CAD build for the part. Positions are in the model's coordinates, mm. Face numbers are marked on the shaded views. Coordinates: 2 decimals unless noted, no trailing zeros. Order: outer loops, then holes, each group sorted by start corner. A loop starts at its lowest first (then second) coordinate and runs counter-clockwise, first axis right, second up. Notation, with made-up numbers: M -11.75,16 L 15.25,16 A20 ccw 15.25,42 Z; hole C 49.25,78 d2. An arc over 180 degrees is marked long. One line per item, written item: value.
from build123d import *

# Parameters (mm, degrees)
SKETCH_W             = 34.6
SKETCH_H             = 24.6
PAD001_DEPTH         = 1
SKETCH002_R          = 1.016
PAD002_DEPTH         = 5
LINEARPATTERN_COUNT  = 2
LINEARPATTERN_PITCH  = 17.9
SKETCH003_W          = 35.8
SKETCH003_H          = 25.8
PAD003_DEPTH         = 10
POCKET_DEPTH         = 12.901
POCKET_DEPTH_BACK    = 12.901
POCKET001_DEPTH      = 17.901
POCKET001_DEPTH_BACK = 17.901
SKETCH006_W          = 34.6
SKETCH006_H          = 24.6
POCKET002_DEPTH      = 2


with BuildPart() as digit001:
    # Sketch → Pad001 (new body)
    with BuildSketch(Plane.XY):
        Rectangle(SKETCH_W, SKETCH_H)
    extrude(amount=PAD001_DEPTH)

    # Sketch002 → Pad002 (join)
    with BuildSketch(Plane.XY):
        with Locations((-2.484719, -9.134)):
            Circle(SKETCH002_R)
        Polygon((-11.875322, 9.261), (-10.815853, 10.15), (-3.50471, 10.15), (-2.75875, 9.261), (-3.818219, 8.372), (-11.129362, 8.372), align=None)
        Polygon((-12.171581, 9.021337), (-11.425621, 8.132337), (-12.643997, 1.222585), (-13.703466, 0.333585), (-14.449425, 1.222585), (-13.23105, 8.132337), align=None)
        Polygon((-2.56357, 8.927415), (-3.623039, 8.038415), (-4.841415, 1.128663), (-4.095455, 0.239663), (-3.035986, 1.128663), (-1.81761, 8.038415), align=None)
        Polygon((-12.448817, 0.889), (-13.508286, 0), (-12.762326, -0.889), (-5.451183, -0.889), (-4.391714, 0), (-5.137674, 0.889), align=None)
        Polygon((-13.804545, -0.239663), (-14.864014, -1.128663), (-16.08239, -8.038415), (-15.33643, -8.927415), (-14.276961, -8.038415), (-13.058585, -1.128663), align=None)
        Polygon((-4.196534, -0.333585), (-5.256003, -1.222585), (-6.474379, -8.132337), (-5.728419, -9.021337), (-4.66895, -8.132337), (-3.450575, -1.222585), align=None)
        Polygon((-15.14125, -9.261), (-14.081781, -8.372), (-6.770638, -8.372), (-6.024678, -9.261), (-7.084147, -10.15), (-14.39529, -10.15), align=None)
    pad002 = extrude(amount=PAD002_DEPTH)

    # LinearPattern: Pad002 ×2
    with Locations(*[(i * LINEARPATTERN_PITCH, 0, 0) for i in range(1, LINEARPATTERN_COUNT)]):
        add(pad002)


with BuildPart() as digit001_1:
    # Body001 placement: moved
    add(digit001.part.moved(Location((0, 0, 5))))


with BuildPart() as obj1:
    # Sketch003 → Pad003 (new body)
    with BuildSketch(Plane.XY):
        Rectangle(SKETCH003_W, SKETCH003_H)
    extrude(amount=PAD003_DEPTH)

    # Sketch004 → Pocket (cut, two sides)
    with BuildSketch(Plane.XZ) as pocket_sk:
        Polygon((-16.9, 0), (-15.9, 1), (15.9, 1), (16.9, 0), align=None)
    extrude(amount=-POCKET_DEPTH, mode=Mode.SUBTRACT)
    extrude(pocket_sk.sketch, amount=POCKET_DEPTH_BACK, mode=Mode.SUBTRACT)

    # Sketch005 → Pocket001 (cut, two sides)
    with BuildSketch(Plane.YZ) as pocket001_sk:
        Polygon((-11.9, 0), (11.9, 0), (10.9, 1), (-10.9, 1), align=None)
    extrude(amount=-POCKET001_DEPTH, mode=Mode.SUBTRACT)
    extrude(pocket001_sk.sketch, amount=POCKET001_DEPTH_BACK, mode=Mode.SUBTRACT)

    # Sketch006 → Pocket002 (cut)
    with BuildSketch(Plane.XY):
        Rectangle(SKETCH006_W, SKETCH006_H)
    extrude(amount=POCKET002_DEPTH, mode=Mode.SUBTRACT)

    # Cut: cut Digit001
    add(digit001_1.part, mode=Mode.SUBTRACT)


solid = obj1.part
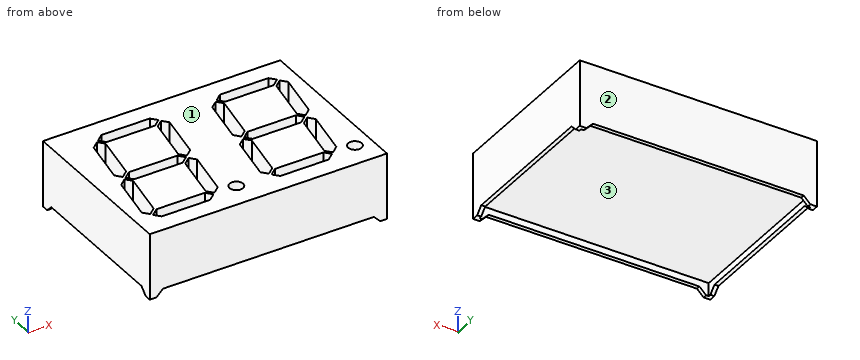
Q1. Slice it at B-B (x = 0). List the corners of the cut face in (y, z), plus the area to 3 significant figures.
Recorded:
outline: M -12.9,1 L -12.3,1 L -12.3,2 L 12.3,2 L 12.3,1 L 12.9,1 L 12.9,10 L -12.9,10 Z; hole M -12.3,5 L 12.3,5 L 12.3,6 L -12.3,6 Z
area: 183 mm^2
Q2. Slice it at A-A (z = 0.5). List the corners of the cut face in (x, y), plus the area to 3 significant figures.
Recorded:
outline: M -17.9,-12.9 L -16.4,-12.9 L -16.4,-12.3 L -17.3,-12.3 L -17.3,-11.4 L -17.9,-11.4 Z; M -17.9,11.4 L -17.3,11.4 L -17.3,12.3 L -16.4,12.3 L -16.4,12.9 L -17.9,12.9 Z; M 16.4,-12.9 L 17.9,-12.9 L 17.9,-11.4 L 17.3,-11.4 L 17.3,-12.3 L 16.4,-12.3 Z; M 16.4,12.3 L 17.3,12.3 L 17.3,11.4 L 17.9,11.4 L 17.9,12.9 L 16.4,12.9 Z
area: 5.76 mm^2
Q3. Pin check, flat tip, straight feed: pin 1 Ø12 at (x, y) = (-3.5, 3.5) entering from -Z. Stop position of the tip, or through.
Recorded:
pin 1: stops at z = 2
Q4. Slice it at D-D (z = 7.75). Give the number of separate pieces and of enclosed holes in the cut face, plus the area to 3 significant figures.
Recorded:
separate pieces: 1
enclosed holes: 16
area: 717 mm^2
Q5. Mould opens along Y. For the marked faces 1, 2 and 3 say: released by +Y, released by -Y, zero draft, split by the parting line, or undercut.
Recorded:
face 1: zero draft
face 2: released by +Y
face 3: undercut
Q6. Drill centre lines: line 1 along Y through (x, z) = (10, 7); line 2 along Z through (x, y) = (11, 4.75); line 3 along X through (y, z) = (3, 9). Where is each one in solid material? Low to high.
Recorded:
line 1: y = -12.9 to -10.15, -8.37 to -0.89, 0.89 to 8.37, 10.15 to 12.9
line 2: z = 2 to 5, 6 to 10
line 3: x = -17.9 to -14.14, -12.33 to -4.51, -2.71 to 3.76, 5.57 to 13.39, 15.19 to 17.9
Q7. Slice it at C-C (y = 2.75). List the corners of the cut face in (x, z).
Recorded:
outline: M -17.9,1 L -17.3,1 L -17.3,2 L 17.3,2 L 17.3,1 L 17.9,1 L 17.9,10 L 15.15,10 L 15.15,6 L 17.3,6 L 17.3,5 L -17.3,5 L -17.3,6 L -14.18,6 L -14.18,10 L -17.9,10 Z; M -12.37,6 L -4.56,6 L -4.56,10 L -12.37,10 Z; M -2.75,6 L 3.72,6 L 3.72,10 L -2.75,10 Z; M 5.53,6 L 13.34,6 L 13.34,10 L 5.53,10 Z
